For this review, take the finished solid that the model builds, in its own axes (mm). Face numbers are marked on the shaded views. A direction names the side the tool comes from. Coordinates: 2 decimals unless noted, no trailing zeros. Loops run counter-clockwise (first coordinate to the right, second up) from the corner with the lowest first, then second, coordinate; pieces in that order, holes last.
1. Take a section at A-A, the plane z = 28. State the section outline as (x, y) points.
2. Machinability: for the marked faces 1, 2 and 3, which of the approach directions +Z, -Z, +X, -X, +Y, -Y give a long, thin tool a straight path to every point of the face, cutting with its end or side? Answer none if there is none.
3. Clearance check with flat-ended pins moving along their axes: P1, Ø5.5, axis at x = -15, y = -3.5, coming from the +Z side; P2, Ø3, axis at y = -2, z = 46.5, coming from the +X side; P3, Ø2, axis at y = -12.5, z = 14, coming from the +X side. State where each tip first meets the part, or that it passes through.
4. Take a section at D-D, the plane z = 46. State the section outline as (x, y) points, then the cut area to 3 significant figures.
5. Take a section at C-C, the plane y = 0. Count the separate pieces of the cut face and the enclosed holes in it, then the cut area to 3 significant figures.
6. Mouldability with a two-part tool opening along Z and no side actions: class the marked faces 4, 5 and 6 as pulls with the +Z half, pulls with the -Z half, needs draft (parallel to the pull), parting line crosses it, or undercut.
7. Take a section at B-B, the plane x = 15.5. State the section outline as (y, z) points.
8. To check wall thickness, follow probe 1 along Z at (x, y) = (17, 15); probe 2 along Y at (x, z) = (26, 53.5); probe 3 along X at (y, z) = (1.5, 38.5). State the ranges of each line that lie inside material, in increasing order.
```python
from build123d import *

# Parameters (mm, degrees)
SKETCH1_R           = 7.5
BOSS_EXTRUDE1_DEPTH = 56
CUT_EXTRUDE1_DEPTH  = 38
SKETCH3_R           = 7
CUT_EXTRUDE2_DEPTH  = 26
CUT_EXTRUDE3_DEPTH  = 6
CUT_EXTRUDE4_DEPTH  = 6


with BuildPart() as part:
    # Sketch1 → Boss-Extrude1 (new body)
    with BuildSketch(Plane.XY):
        with BuildLine():
            Line((-28, -19), (31, -19))
            Line((31, -19), (46, -10.339745962))
            Line((46, -10.339745962), (46, 10.339745962))
            Line((46, 10.339745962), (31, 19))
            Line((31, 19), (6.698703146, 19))
            ThreePointArc((6.698703146, 19), (-12.009583788, 15.368092477), (-28, 5))
            Line((-28, 5), (-28, -19))
        make_face()
        Circle(SKETCH1_R, mode=Mode.SUBTRACT)
    extrude(amount=BOSS_EXTRUDE1_DEPTH)

    # Sketch2 → Cut-Extrude1 (cut)
    with BuildSketch(Plane(origin=(0, 19, 0), x_dir=(1, 0, 0), z_dir=(0, 1, 0))):
        Polygon((31, 0), (46, -15), (46, 0), align=None)
        Polygon((31, -56), (46, -41), (46, -56), align=None)
        Polygon((-28, -8), (-12, -8), (-12, -14), (20, -14), (20, -42), (-12, -42), (-12, -48), (-28, -48), align=None)
    extrude(amount=-CUT_EXTRUDE1_DEPTH, mode=Mode.SUBTRACT)

    # Sketch3 → Cut-Extrude2 (cut)
    with BuildSketch(Plane(origin=(46, 0, 0), x_dir=(0, 0, -1), z_dir=(1, 0, 0))):
        with Locations((-28, 0)):
            Circle(SKETCH3_R)
    extrude(amount=-CUT_EXTRUDE2_DEPTH, mode=Mode.SUBTRACT)

    # Sketch7 → Cut-Extrude3 (cut)
    with BuildSketch(Plane.XY.offset(56)):
        with BuildLine():
            Line((-28, 2.166247904), (-28, -17))
            Line((-28, -17), (29, -17))
            Line((29, -17), (29, 17))
            Line((29, 17), (6.698703146, 17))
            ThreePointArc((6.698703146, 17), (-12.169525449, 13.136039125), (-28, 2.166247904))
        make_face()
    extrude(amount=-CUT_EXTRUDE3_DEPTH, mode=Mode.SUBTRACT)

    # Sketch10 → Cut-Extrude4 (cut)
    with BuildSketch(Plane.XY.offset(50)):
        with BuildLine():
            Line((-10, -17), (-10, 14.001703448))
            ThreePointArc((-10, 14.001703448), (-1.784168847, 16.244479918), (6.698703146, 17))
            Line((6.698703146, 17), (29, 17))
            Line((29, 17), (29, -17))
            Line((29, -17), (-10, -17))
        make_face()
    extrude(amount=-CUT_EXTRUDE4_DEPTH, mode=Mode.SUBTRACT)


solid = part.part
```
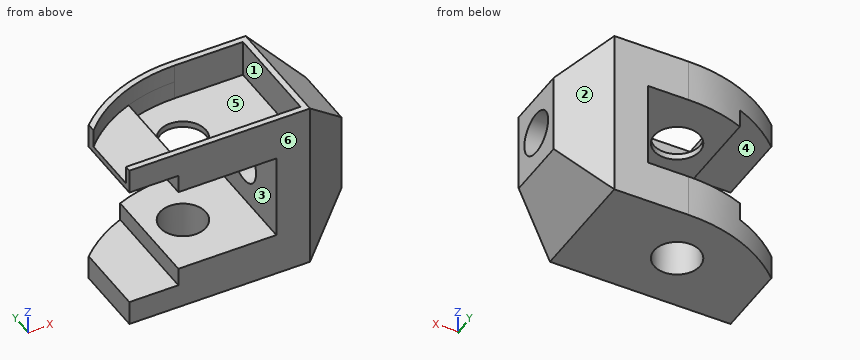
Results list:
1. outline: (20, -19) - (31, -19) - (46, -10.34) - (46, -7) - (20, -7) - close; (20, 7) - (46, 7) - (46, 10.34) - (31, 19) - (20, 19) - close
2. face 1: +Z
2. face 2: +Z, -Z, +X, +Y
2. face 3: -X, +Y, -Y
3. P1: stops at z = 50
3. P2: stops at x = 42
3. P3: stops at x = 43.99
4. outline: (-12, -19) - (31, -19) - (41, -13.23) - (41, 13.23) - (31, 19) - (6.7, 19) arc R50 ccw to (-12, 15.37) - close; hole (-10, -17) - (29, -17) - (29, 17) - (6.7, 17) arc R48 ccw to (-10, 14) - close
4. area: 624 mm2
5. separate pieces: 4
5. enclosed holes: 0
5. area: 1,200 mm2
6. face 4: undercut
6. face 5: pulls with the +Z half
6. face 6: needs draft
7. outline: (-19, 0) - (19, 0) - (19, 14) - (-19, 14) - close; (-19, 42) - (19, 42) - (19, 56) - (17, 56) - (17, 44) - (-17, 44) - (-17, 56) - (-19, 56) - close
8. probe 1: z = 0 to 14, 42 to 44
8. probe 2: y = -19 to -17, 17 to 19
8. probe 3: x = 20 to 46
